```python
from build123d import *

# Parameters (mm, degrees)
F0_R        = 36.3127781595
F1_DEPTH    = 76.2
F0_R_2      = 55.3433829245
F2_DEPTH    = 50.8
F0_R_3      = 72.7478178249
F3_DEPTH    = 25.4
F4_SIZE     = 25.39999
F5_S5_R     = 55.3433829245
F5_T6_DEPTH = 105


# Not quite as in the source:
# - a fillet or chamfer that OpenCascade refuses, or shapes differently, is made with other operations: its cross-section is extruded or revolved along the edge and cut away or added
# - a fillet or chamfer is up to 0.001 mm smaller than in the source, because OpenCascade refuses the exact size


with BuildPart() as f1:
    # F0 (on Top) → F1 (new body)
    with BuildSketch(Plane.XY):
        Circle(F0_R)
    extrude(amount=F1_DEPTH)

    # F0 (on Top) → F2 (join)
    with BuildSketch(Plane.XY):
        Circle(F0_R_2)
        Circle(F0_R, mode=Mode.SUBTRACT)
    extrude(amount=F2_DEPTH)

    # F0 (on Top) → F3 (join)
    with BuildSketch(Plane.XY):
        Circle(F0_R_3)
        Circle(F0_R_2, mode=Mode.SUBTRACT)
    extrude(amount=F3_DEPTH)

    # F4 (size 25.4 in the source; OpenCascade refuses exactly that, so slightly less here)
    f4_edges = [f1.edges().sort_by_distance(p)[0] for p in [
        (-36.312778, 0, 76.2),
    ]]
    chamfer(f4_edges, length=F4_SIZE)

    # F5: chamfer of 18.542 on 2 edges, made by hand


with BuildPart() as f5_tool2:
    # F5_s3 → F5_t4 (revolve)
    with BuildSketch(Plane.XZ):
        Polygon((54.2058178249, 25.4), (72.7478178249, 6.858), (72.7478178249, 25.4), align=None)
    revolve(axis=Axis((0, 0, 25.4), (0, 0, 1)))

    # F5_s5 → F5_t6 (cut, symmetric)
    with BuildSketch(Plane.XY.offset(16.1)):
        Circle(F5_S5_R)
    extrude(amount=F5_T6_DEPTH, both=True, mode=Mode.SUBTRACT)


with BuildPart() as f1_1:
    add(f1.part)

    # F5_t1: cut F5_tool2
    add(f5_tool2.part, mode=Mode.SUBTRACT)

    # F5_s7 → F5_t8 (revolve, cut)
    with BuildSketch(Plane.XZ):
        Polygon((36.8013829245, 50.8), (55.3433829245, 32.258), (55.3433829245, 50.8), align=None)
    revolve(axis=Axis((0, 0, 50.8), (0, 0, 1)), mode=Mode.SUBTRACT)

    # F6: fillet of radius 25.4 on 4 edges, made by hand

    # F6_s1 → F6_t2 (revolve, cut)
    with BuildSketch(Plane.XZ):
        with BuildLine():
            ThreePointArc((18.3522759174, 68.7605122421), (10.1119228573, 74.2665401258), (0.3917636752, 76.2))
            Line((0.3917636752, 76.2), (0.3917636752, 76.708))
            Line((0.3917636752, 76.708), (11.1232086492, 76.708))
            Line((11.1232086492, 76.708), (18.7114861622, 69.119722487))
            Line((18.7114861622, 69.119722487), (18.3522759174, 68.7605122421))
        make_face()
    revolve(axis=Axis((0, 0, 76.2), (0, 0, 1)), mode=Mode.SUBTRACT)

    # F6_s3 → F6_t4 (revolve, cut)
    with BuildSketch(Plane.XZ):
        with BuildLine():
            ThreePointArc((48.0441667783, 39.5572161462), (53.0070025329, 32.5365446991), (55.3433829245, 24.2624349004))
            Line((55.3433829245, 24.2624349004), (55.8485774923, 24.3157495203))
            ThreePointArc((55.8485774923, 24.3157495203), (55.8513829245, 28.2602174502), (55.8513829245, 32.258))
            Line((55.8513829245, 32.258), (55.7025931693, 32.6172102448))
            Line((55.7025931693, 32.6172102448), (48.4033770231, 39.9164263911))
            Line((48.4033770231, 39.9164263911), (48.0441667783, 39.5572161462))
        make_face()
    revolve(axis=Axis((0, 0, 32.258), (0, 0, 1)), mode=Mode.SUBTRACT)

    # F6_s5 → F6_t6 (revolve, cut)
    with BuildSketch(Plane.XZ):
        with BuildLine():
            ThreePointArc((65.6214802199, 13.984337605), (70.2919041112, 7.5564195951), (72.7478178249, 0))
            Line((72.7478178249, 0), (73.2495548219, 0.0795234927))
            ThreePointArc((73.2495548219, 0.0795234927), (73.2558178249, 3.429), (73.2558178249, 6.858))
            Line((73.2558178249, 6.858), (73.1070280697, 7.2172102448))
            Line((73.1070280697, 7.2172102448), (65.9806904647, 14.3435478499))
            Line((65.9806904647, 14.3435478499), (65.6214802199, 13.984337605))
        make_face()
    revolve(axis=Axis((0, 0, 6.858), (0, 0, 1)), mode=Mode.SUBTRACT)

    # F6_s7 → F6_t8 (revolve, cut)
    with BuildSketch(Plane.XZ):
        with BuildLine():
            ThreePointArc((36.3127781595, 50.8), (37.9669911758, 49.5120321576), (39.5093522451, 48.0920306794))
            Line((39.5093522451, 48.0920306794), (39.86856249, 48.4512409242))
            Line((39.86856249, 48.4512409242), (37.1605931693, 51.1592102448))
            Line((37.1605931693, 51.1592102448), (36.8013829245, 51.308))
            ThreePointArc((36.8013829245, 51.308), (36.557080542, 51.308), (36.6080569226, 51.2133696313))
            Line((36.6080569226, 51.2133696313), (36.3127781595, 50.8))
        make_face()
    revolve(axis=Axis((0, 0, 50.8), (0, 0, 1)), mode=Mode.SUBTRACT)


solid = f1_1.part
```
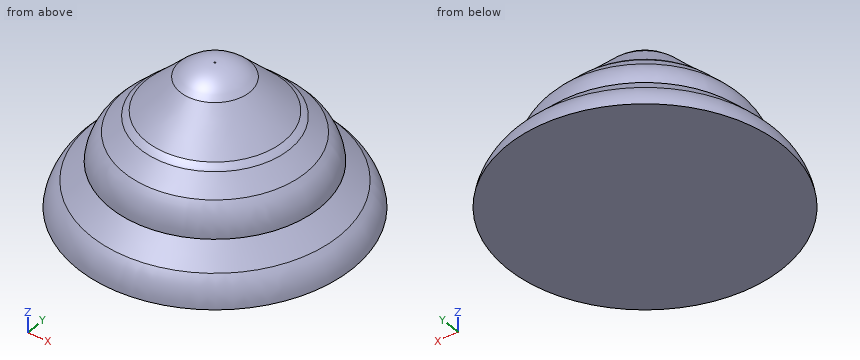
Build history of the part. All positions in model axes, mm. Coordinates: 2 decimals unless noted, no trailing zeros. Order: outer loops, then holes, each group sorted by start corner. A loop starts at its lowest first (then second) coordinate and runs counter-clockwise, first axis right, second up. Notation, with made-up numbers: (-22, 49) -> (31, 49) arc R14 ccw to (31, 55) -> close; hole circle Ø10 at (-35, 12.25). An arc over 180 degrees is marked (long way). Answer in a Markdown table with one row per item. Add a question column.
Q1. Wall check: line 1 along Z through (x, y) = (2, -13); line 2 along Z through (x, y) = (32, 9); line 3 along X through (y, z) = (-11, 27). Give the ranges that are in metal, low to high. Write a range as [from, to].
Q2. Drop flat-ended pins along their axis: pin 1 (4 mm diameter, centred on x = 20, z = 64, fed in from -Y); pin 2 (1.5 mm diameter, centred on y = -20.5, z = 56.5, fed in from -X); pin 3 (10 mm diameter, centred on x = 15, z = 63, fed in from -Y). Give the stop position or say it passes through.
Q3. Band-saw the part on B-B, the plane z = 36. List the corners of the cut face in (x, y).
Q4. Band-saw the part on A-A, the plane z = 67. List the corners of the cut face in (x, y), then the cut area to 3 significant figures.
Answers follow:
| question | item | result |
|---|---|---|
| 1 | line 1 | [0, 72.76] |
| 1 | line 2 | [0, 53.87] |
| 1 | line 3 | [-53.79, 53.79] |
| 2 | pin 1 | y = -16.04 |
| 2 | pin 2 | x = -23.92 |
| 2 | pin 3 | y = -25.58 |
| 3 | outline | circle Ø102.01 at (0, 0) |
| 4 | outline | circle Ø40.23 at (0, 0) |
| 4 | area | 1,270 mm^2 |
